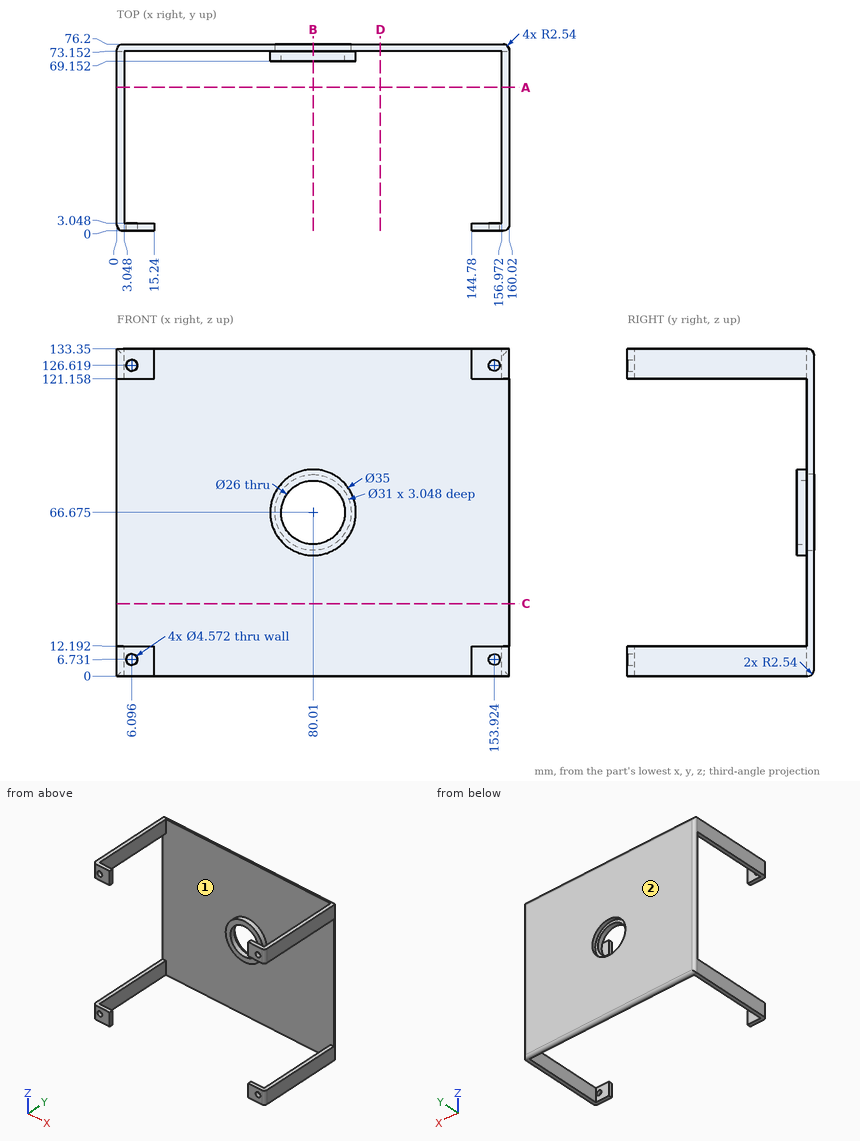
Can you work these out from the drawing? Everything is in mm from the part's minimum corner. Give positions to 0.01 mm unless a question says otherwise; leave off trailing zeros. Loops run counter-clockwise (first coordinate to the right, second up) from the corner with the lowest first, then second, coordinate; pieces in that order, holes last. Notation, with made-up numbers: (28.25, 37.25) - (38.25, 37.25) arc R18 cw to (38.25, 58.25) - close; hole circle Ø1 at (-38.75, 65.5). An arc over 180 degrees is marked (long way). Use one line per item in the form item = value.
1. Thinking about a two-plate mould opening in X: for the marked faces 1 and 2, which applies, released by +X, released by -X, zero draft, split by the parting line, or undercut?
Response values:
face_1 = undercut
face_2 = zero draft
2. I want a section at A-A (y = 58.5). Please give me the cut outline in (x, z).
Response values:
outline = (0, 0) - (3.05, 0) - (3.05, 12.19) - (0, 12.19) - close; (0, 121.16) - (3.05, 121.16) - (3.05, 133.35) - (0, 133.35) - close; (156.97, 0) - (160.02, 0) - (160.02, 12.19) - (156.97, 12.19) - close; (156.97, 121.16) - (160.02, 121.16) - (160.02, 133.35) - (156.97, 133.35) - close
3. I need wall thicknesses on probe 1 along Z at (x, y) = (80, 71) (3 decimals); probe 2 along Y at (x, z) = (112.5, 37); probe 3 along X at (y, z) = (71, 125.5). Which ranges of each line are inside material? Lowest first, please.
Response values:
probe_1 = 49.175 to 53.675, 79.675 to 84.175
probe_2 = 73.15 to 76.2
probe_3 = 0 to 3.05, 156.97 to 160.02
4. I'm going to push flat-ended pins straight in: pin 1 Ø12 at (x, y) = (154, 46.5) entering from +Z; pin 2 Ø10 at (x, z) = (112, 68.5) entering from -Y; pin 3 Ø2.5 at (y, z) = (1, 130.5) entering from +X. Where does each tip first touch, or does it pass through?
Response values:
pin_1 = 133.35
pin_2 = 73.15
pin_3 = 160
5. I want a section at D-D (x = 107.5). Please give me the cut outline in (y, z), and give its area (3 significant figures).
Response values:
outline = (73.15, 0) - (73.66, 0) arc R2.54 ccw to (76.2, 2.54) - (76.2, 130.81) arc R2.54 ccw to (73.66, 133.35) - (73.15, 133.35) - close
area = 404 mm²
6. I want a section at B-B (x = 80.01). Please give me the cut outline in (y, z) (3 decimals).
Response values:
outline = (69.152, 49.175) - (73.152, 49.175) - (73.152, 0) - (73.66, 0) arc R2.54 ccw to (76.2, 2.54) - (76.2, 51.175) - (73.152, 51.175) - (73.152, 53.675) - (69.152, 53.675) - close; (69.152, 79.675) - (73.152, 79.675) - (73.152, 82.175) - (76.2, 82.175) - (76.2, 130.81) arc R2.54 ccw to (73.66, 133.35) - (73.152, 133.35) - (73.152, 84.175) - (69.152, 84.175) - close
7. I want a section at C-C (z = 29.5). Please give me the cut outline in (x, y), and give its area (3 significant figures).
Response values:
outline = (0, 73.15) - (160.02, 73.15) - (160.02, 73.66) arc R2.54 ccw to (157.48, 76.2) - (2.54, 76.2) arc R2.54 ccw to (0, 73.66) - close
area = 485 mm²
